The figure shows three views and two pictorial views of one solid part (mm, origin at its lowest corner). Answer the questions. A direction names the side the tool comes from. Round coordinates to 2 decimals unless told otherwise and drop trailing zeros. Order: outer loops, then holes, each group sorted by start corner. A loop starts at its lowest first (then second) coordinate and runs counter-clockwise, first axis right, second up. Notation, with made-up numbers: M 58.5,-2.75 L 85.5,-2.75 A17 ccw 85.5,7.25 Z; hole C 16.5,65.25 d9. An arc over 180 degrees is marked long. Return JSON: item names as keys, results as strings.
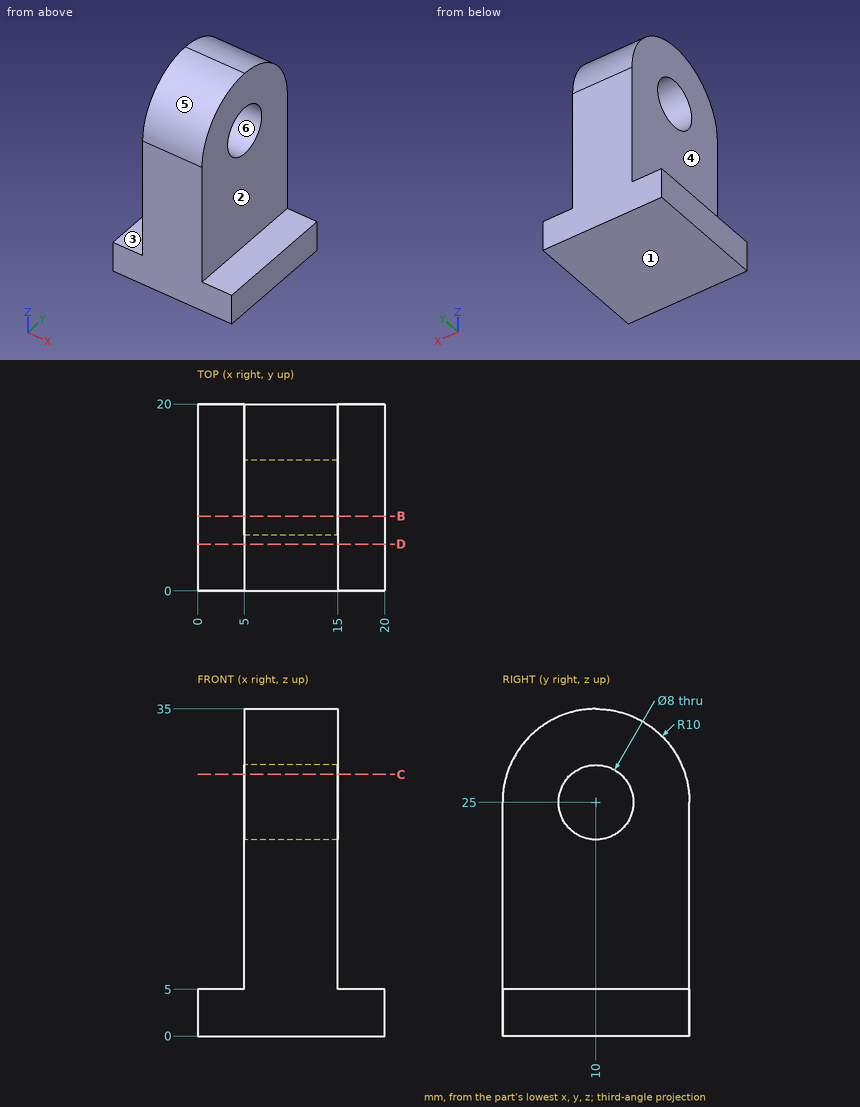
Item 1: Find section D-D (y = 5). Determine the outline of the cut face in (x, z).
Output:
{"outline": "M 0,0 L 20,0 L 20,5 L 15,5 L 15,33.66 L 5,33.66 L 5,5 L 0,5 Z"}
Item 2: Find section B-B (y = 8). Determine the outline of the cut face in (x, z), plus the area to 3 significant figures.
Output:
{"outline": "M 0,0 L 20,0 L 20,5 L 15,5 L 15,21.54 L 5,21.54 L 5,5 L 0,5 Z; M 5,28.46 L 15,28.46 L 15,34.8 L 5,34.8 Z", "area": "329 mm^2"}
Item 3: Each of these flat-tipped pins is pushed along its axis until it touches: pin 1 (1.5 mm diameter, centred on x = 16.5, y = 7.5, fed in from +Z); pin 2 (10 mm diameter, centred on y = 8.5, z = 22, fed in from +X); pin 3 (8 mm diameter, centred on y = 16.5, z = 15, fed in from -X). Where does it stop, or does it pass through?
Output:
{"pin 1": "stops at z = 5", "pin 2": "stops at x = 15", "pin 3": "stops at x = 5"}
Item 4: Which of the six approach directions +Z, -Z, +X, -X, +Y, -Y give full straight-line access (tool end or side, diameter ignored) to the marked faces 1, 2 and 3?
Output:
{"face 1": "-Z, +X, -X, +Y, -Y", "face 2": "+Z, +X, +Y, -Y", "face 3": "+Z, -X, +Y, -Y"}
Item 5: Consider line 1 along Z through (x, y) = (8.25, 10); line 2 along Z through (x, y) = (3.5, 9.75); line 3 along X through (y, z) = (1, 6). Determine where each line is inside the solid, lowest interval first. Write a range as [from, to].
Output:
{"line 1": "z = [0, 21], [29, 35]", "line 2": "z = [0, 5]", "line 3": "x = [5, 15]"}
Item 6: The mould has two halves that part along Y. Classify the marked faces 4, 5 and 6: pulls with the +Y half, pulls with the -Y half, needs draft (parallel to the pull), parting line crosses it, or undercut.
Output:
{"face 4": "needs draft", "face 5": "pulls with the -Y half", "face 6": "undercut"}
Item 7: Find section C-C (z = 28). Determine the outline of the cut face in (x, y).
Output:
{"outline": "M 5,0.46 L 15,0.46 L 15,7.35 L 5,7.35 Z; M 5,12.65 L 15,12.65 L 15,19.54 L 5,19.54 Z"}
